```python
from build123d import *

# Parameters (mm, degrees)
SKETCH2_W                       = 120
SKETCH2_H                       = 50
BOSS_EXTRUDE1_DEPTH             = 15
AUFSATZ_LINEAR_START            = 47.5
AUFSATZ_LINEAR_AUSTRAGEN3_DEPTH = 47.5
SCHNITT_LINEAR_START            = 35
SKIZZE7_R                       = 7.5
SCHNITT_LINEAR_AUSTRAGEN2_DEPTH = 12.5
SCHNITT_LINEAR_START_2          = 10
SKIZZE7_2_R                     = 7.5
SCHNITT_LINEAR_AUSTRAGEN3_DEPTH = 10
SCHNITT_LINEAR_AUSTRAGEN4_REACH = 84.234
SKIZZE8_R                       = 1
SCHNITT_LINEAR_AUSTRAGEN5_DEPTH = 126.77149982
SKIZZE10_R                      = 2
SCHNITT_LINEAR_AUSTRAGEN7_DEPTH = 82.469960946
SPIEGELN3_COPY_1_SKETCH_R       = 2
SPIEGELN3_COPY_1_DEPTH          = 82.469960946
SKIZZE12_R                      = 2
SCHNITT_LINEAR_AUSTRAGEN8_DEPTH = 10


with BuildPart() as part:
    # Sketch2 → Boss-Extrude1 (new body)
    with BuildSketch(Plane(origin=(0, 0, 0), x_dir=(1, 0, 0), z_dir=(0, 1, 0))):
        with Locations((13.101876656, 9.54663752)):
            Rectangle(SKETCH2_W, SKETCH2_H)
    extrude(amount=BOSS_EXTRUDE1_DEPTH)

    # Sketch3 → Cut-Revolve8 (revolve, cut)
    with BuildSketch(Plane(origin=(0, 0, 0), x_dir=(1, 0, 0), z_dir=(0, 1, 0))):
        Polygon((63.101876656, 9.54663752), (63.101876656, 17.04663752), (3.101876656, 17.04663752), (3.101876656, 19.54663752), (-36.898123344, 19.54663752), (-36.898123344, 9.54663752), align=None)
    revolve(axis=Axis((74.354835368, 0, -9.54663752), (-1, 0, 0)), mode=Mode.SUBTRACT)

    # Skizze2 → Aufsatz-Linear austragen3 (add)
    with BuildSketch(Plane.ZY.offset(-63.101876656).offset(AUFSATZ_LINEAR_START)):
        with BuildLine():
            Line((-3.54663752, 0), (-2.04663752, 0))
            ThreePointArc((-2.04663752, 0), (-2.491532858, 2.544700024), (-3.773437043, 4.7875))
            Line((-3.773437043, 4.7875), (-4.928077138, 3.83))
            ThreePointArc((-4.928077138, 3.83), (-3.902553791, 2.035760019), (-3.54663752, 0))
        make_face()
    aufsatz_linear_austragen3 = extrude(amount=-AUFSATZ_LINEAR_AUSTRAGEN3_DEPTH)

    # Spiegeln1: Aufsatz-Linear austragen3 across plane
    add(aufsatz_linear_austragen3.mirror(Plane.XY.offset(-9.54663752)))

    # Skizze7 → Schnitt-Linear austragen2 (cut)
    with BuildSketch(Plane.ZY.offset(-63.101876656).offset(SCHNITT_LINEAR_START)):
        with Locations((-9.54663752, 0)):
            Circle(SKIZZE7_R)
    extrude(amount=-SCHNITT_LINEAR_AUSTRAGEN2_DEPTH, mode=Mode.SUBTRACT)

    # Skizze7<2> → Schnitt-Linear austragen3 (cut)
    with BuildSketch(Plane.ZY.offset(-63.101876656).offset(SCHNITT_LINEAR_START_2)):
        with Locations((-9.54663752, 0)):
            Circle(SKIZZE7_2_R)
    extrude(amount=-SCHNITT_LINEAR_AUSTRAGEN3_DEPTH, mode=Mode.SUBTRACT)

    # Skizze8 → Schnitt-Linear austragen4 (cut, up to next)
    with BuildSketch(Plane(origin=(0, 15, 0), x_dir=(1, 0, 0), z_dir=(0, 1, 0)), mode=Mode.PRIVATE) as schnitt_linear_austragen4_sk1:
        with Locations(Location((58.101876656, 9.54663752, 0), (0, 0, 270))):
            Circle(SKIZZE8_R)
    schnitt_linear_austragen4_tool1 = extrude(schnitt_linear_austragen4_sk1.sketch, amount=-SCHNITT_LINEAR_AUSTRAGEN4_REACH, mode=Mode.PRIVATE) & part.part
    # Skizze8 → Schnitt-Linear austragen4 (cut, up to next)
    with BuildSketch(Plane(origin=(0, 15, 0), x_dir=(1, 0, 0), z_dir=(0, 1, 0)), mode=Mode.PRIVATE) as schnitt_linear_austragen4_sk2:
        with Locations(Location((34.351876656, 9.54663752, 0), (0, 0, 270))):
            Circle(SKIZZE8_R)
    schnitt_linear_austragen4_tool2 = extrude(schnitt_linear_austragen4_sk2.sketch, amount=-SCHNITT_LINEAR_AUSTRAGEN4_REACH, mode=Mode.PRIVATE) & part.part
    # Skizze8 → Schnitt-Linear austragen4 (cut, up to next)
    with BuildSketch(Plane(origin=(0, 15, 0), x_dir=(1, 0, 0), z_dir=(0, 1, 0)), mode=Mode.PRIVATE) as schnitt_linear_austragen4_sk3:
        with Locations(Location((-16.898123344, 9.54663752, 0), (0, 0, 270))):
            Circle(SKIZZE8_R)
    schnitt_linear_austragen4_tool3 = extrude(schnitt_linear_austragen4_sk3.sketch, amount=-SCHNITT_LINEAR_AUSTRAGEN4_REACH, mode=Mode.PRIVATE) & part.part
    add(schnitt_linear_austragen4_tool1.solids().sort_by_distance((58.101877, 15, -9.546638))[0], mode=Mode.SUBTRACT)
    add(schnitt_linear_austragen4_tool2.solids().sort_by_distance((34.351877, 15, -9.546638))[0], mode=Mode.SUBTRACT)
    add(schnitt_linear_austragen4_tool3.solids().sort_by_distance((-16.898123, 15, -9.546638))[0], mode=Mode.SUBTRACT)

    # Skizze9 → Schnitt-Linear austragen5 (cut, through all)
    with BuildSketch(Plane.ZY.offset(46.898123344)):
        Polygon((-34.54663752, 5), (-22.04663752, 5), (-22.04663752, 15), (2.95336248, 15), (2.95336248, 5), (15.45336248, 5), (15.45336248, 15), (-34.54663752, 15), align=None)
    extrude(amount=-SCHNITT_LINEAR_AUSTRAGEN5_DEPTH, mode=Mode.SUBTRACT)

    # Skizze10 → Schnitt-Linear austragen7 (cut, through all)
    with BuildSketch(Plane(origin=(0, 5, 0), x_dir=(1, 0, 0), z_dir=(0, 1, 0))):
        with Locations(Location((65.601876656, 27.04663752, 0), (0, 0, 270))):
            Circle(SKIZZE10_R)
    schnitt_linear_austragen7 = extrude(amount=-SCHNITT_LINEAR_AUSTRAGEN7_DEPTH, mode=Mode.SUBTRACT)

    # Spiegeln2: Schnitt-Linear austragen7 across plane
    add(schnitt_linear_austragen7.mirror(Plane.XY.offset(-9.54663752)), mode=Mode.SUBTRACT)

    # Spiegeln3: Schnitt-Linear austragen7 across plane
    add(schnitt_linear_austragen7.mirror(Plane(origin=(13.101876656, 0, 0), x_dir=(0, 0, 1), z_dir=(1, 0, 0))), mode=Mode.SUBTRACT)

    # Spiegeln3 copy 1 sketch → Spiegeln3 copy 1 (cut, through all)
    with BuildSketch(Plane(origin=(26.203753312, 5, -19.09327504), x_dir=(-1, 0, 0), z_dir=(0, 1, 0))):
        with Locations(Location((65.601876656, 27.04663752, 0), (0, 0, 270))):
            Circle(SPIEGELN3_COPY_1_SKETCH_R)
    extrude(amount=-SPIEGELN3_COPY_1_DEPTH, mode=Mode.SUBTRACT)

    # Skizze12 → Schnitt-Linear austragen8 (cut)
    with BuildSketch(Plane(origin=(0, 5, 0), x_dir=(1, 0, 0), z_dir=(0, 1, 0))):
        with Locations(Location((13.101876656, 27.04663752, 0), (0, 0, 270))):
            Circle(SKIZZE12_R)
        with Locations(Location((13.101876656, -7.95336248, 0), (0, 0, 270))):
            Circle(SKIZZE12_R)
    extrude(amount=-SCHNITT_LINEAR_AUSTRAGEN8_DEPTH, mode=Mode.SUBTRACT)


solid = part.part
```
Part model, mm, in its own coordinate system. A direction names the side the tool comes from. Coordinates: 2 decimals unless noted, no trailing zeros. Order: outer loops, then holes, each group sorted by start corner. A loop starts at its lowest first (then second) coordinate and runs counter-clockwise, first axis right, second up. Notation, with made-up numbers: (23.25, 20.5) -> (32.25, 20.5) arc R25 cw to (32.25, 32.5) -> close; hole circle Ø7 at (-15, 40.5). An arc over 180 degrees is marked (long way). Put each result on its own line as item: value. Start each with the question number.
(1) Pin check, flat tips, straight feed: pin 1 Ø13.5 at (x, z) = (29.5, -30) entering from +Y; pin 2 Ø1.5 at (x, y) = (-14.5, 11.5) entering from +Z; pin 3 Ø2.5 at (x, z) = (58.1, -9.55) entering from -Y; pin 4 Ø1.5 at (y, z) = (7.5, 6.5) entering from -X. Stop position of each tip, or through.
(2) Mould opens along Z. For faces 1 (the face through (12, 0, -20)), 2 (the face through (21.76, 2.06, -3.91)), 3 (the face through (12, 10, -22.047)) say: pulls with the +Z half, pulls with the -Z half, needs draft (parallel to the pull), parting line crosses it, or undercut.
(3) Band-saw the part on B-B (x = 30.5). Give the cut face in (y, z).
(4) Which spindle directions (+Z, -Z, +X, -X, +Y, -Y) get a long thin tool onto all of the face, cutting with end or side? Do faces 4 (the face through (57.126, 11.269, -9.763)), 5 (the face through (12, 5, -30)), 6 (the face through (53.102, 2, -16)). Say none if no direction does.
(5) Probe line 1 along X through (y, z) = (1, -11); line 2 along Z through (x, y) = (10.5, 0.5); line 3 along Z through (x, y) = (-21, 8). List the from-to ranges inside material, lowest first. Write a range as [from, to].
(6) Band-saw the part on A-A (x = -29). Give the cut face in (y, z), then the cut area to 3 significant figures.
Determined:
1. pin 1: stops at y = 5
1. pin 2: stops at z = 2.95
1. pin 3: stops at y = 7.39
1. pin 4: passes through
2. face 1: needs draft
2. face 2: undercut
2. face 3: pulls with the -Z half
3. outline: (0, -34.55) -> (5, -34.55) -> (5, -22.05) -> (15, -22.05) -> (15, 2.95) -> (5, 2.95) -> (5, 15.45) -> (0, 15.45) -> (0, -2.05) arc R7.5 cw to (0, -17.05) -> close
4. face 4: +Y, -Y
4. face 5: -Z, +X, -X, +Y
4. face 6: -Y
5. line 1: x = [-46.9, -36.9], [63.1, 73.1]
5. line 2: z = [-34.55, -17.03], [-2.06, 15.45]
5. line 3: z = [-22.05, -15.55], [-3.55, 2.95]
6. outline: (0, -34.55) -> (5, -34.55) -> (5, -22.05) -> (15, -22.05) -> (15, 2.95) -> (5, 2.95) -> (5, 15.45) -> (0, 15.45) -> (0, 0.45) arc R10 cw to (0, -19.55) -> close
6. area: 343 mm²
